from build123d import *

# Parameters (mm, degrees)
F0_W        = 50
F0_H        = 50
F1_DEPTH    = 35
F3_D        = 25
F4_T1_DEPTH = 116.8637576871
F5_T1_DEPTH = 116.8637576871
F6_DEPTH    = 20
F7_T1_DEPTH = 75.7168298797
F10_DEPTH   = 5
F12_DEPTH   = 5


# Not quite as in the source:
# - a fillet or chamfer that OpenCascade refuses, or shapes differently, is made with other operations: its cross-section is extruded or revolved along the edge and cut away or added
# - two fillets or chamfers of one size are made in one step


with BuildPart() as f1:
    # F0 (on Top) → F1 (new body)
    with BuildSketch(Plane.XY):
        with Locations((25, 25)):
            Rectangle(F0_W, F0_H)
    extrude(amount=F1_DEPTH)

    # F3 (through all)
    with Locations(Plane.XZ):
        with Locations((25, 21.1336053908)):
            Hole(F3_D / 2)

    # F4: chamfer of 13 on 1 edges, made by hand

    # F4_s2 → F4_t1 (cut)
    with BuildSketch(Plane.YZ.offset(-33.4318788436)):
        Polygon((0, 22), (13, 35), (0, 35), align=None)
    extrude(amount=F4_T1_DEPTH, mode=Mode.SUBTRACT)

    # F5: chamfer of 13 on 1 edges, made by hand

    # F5_s2 → F5_t1 (cut)
    with BuildSketch(Plane.YZ.offset(-33.4318788436)):
        Polygon((37, 35), (50, 22), (50, 35), align=None)
    extrude(amount=F5_T1_DEPTH, mode=Mode.SUBTRACT)

    # F6 (add): a face of the model
    f6_faces = [f1.faces().sort_by_distance(p)[0] for p in [
        (25, 25, 35),
    ]]
    extrude(f6_faces, amount=F6_DEPTH)

    # F7: chamfer of 5 on 4 edges, made by hand

    # F7_s2 → F7_t1 (cut)
    with BuildSketch(Plane.YZ.offset(-12.8584149398)):
        Polygon((13, 50), (18, 55), (13, 55), align=None)
        Polygon((37, 50), (32, 55), (37, 55), align=None)
    extrude(amount=F7_T1_DEPTH, mode=Mode.SUBTRACT)

    # F9 (on face) → F10 (join)
    with BuildSketch(Plane.YZ.offset(50)):
        Polygon((13, 50), (13, 35), (37, 35), (37, 50), (32, 55), (18, 55), align=None)
    extrude(amount=F10_DEPTH)

    # F11 (on face) → F12 (join)
    with BuildSketch(Plane(origin=(0, 0, 0), x_dir=(0, -1, 0), z_dir=(-1, 0, 0))):
        Polygon((-37, 50), (-37, 35), (-13, 35), (-13, 50), (-18, 55), (-32, 55), align=None)
    extrude(amount=F12_DEPTH)


solid = f1.part
Verification items for the finished model (mm, model axes). A direction names the side the tool comes from. Coordinates: 2 decimals unless noted, no trailing zeros. Write each loop counter-clockwise with the first axis right and the second up, starting at its lowest first coordinate (ties: lowest second). Pieces come first, ordered by that corner, then holes. Notation, with made-up numbers: (-25.5, -21) -> (-4.5, -21) arc R20 ccw to (-4.5, -12) -> close; hole circle Ø4 at (43.5, -31.5). An arc over 180 degrees is marked (long way). One line per item, written item: value. Start each with the question number.
Q1. Mould release check, pull along X, two halves, no side actions. Record for faces 1 (the flat face through (25, 38, 34)), 2 (the flat face through (55, 25, 45)), 3 (the cylindrical face through (28, 25, 9)): pulls with the +X half, pulls with the -X half, needs draft (parallel to the pull), parting line crosses it, or undercut.
Q2. Cross-section at C-C on y = 30. Enter the section's corners in (x, z).
Q3. Cross-section at B-B on x = 25. Enter the section's corners in (y, z).
Q4. Go/stop test with flat-tipped pins: P1, Ø4.5, axis at x = 38.5, z = 41, coming from the -Y side; P2, Ø10.5, axis at y = 13.5, z = 23, coming from the +X side; P3, Ø4, axis at x = 53, y = 27.5, coming from the -Z side; P4, Ø20, axis at x = 25, z = 21.13, coming from the -Y side. Record where each tip stops, or that it passes through.
Q5. Cross-section at A-A on z = 15.5. Enter the section's corners in (x, y), and give its area (3 significant figures).
Q6. Access from +Z, -Z, +X, -X, +Y, -Y to the whole of each face (thin tool, end or side, straight path). Record for faces 4 (the flat face through (25, 13, 42)), 5 (the flat face through (50, 25, 17)), 6 (the flat face through (25, 37, 43)).
Q7. Cross-section at D-D on x = 42. Enter the section's corners in (y, z), and give its area (3 significant figures).
Q8. Thickness scan on L1, parallel to Z at x = 25, y = 28; L2, parallel to X at y = 43, z = 8; L3, parallel to X at y = 14, z = 18. Record the ranges inside material, lowest first. Write a range as from..to.
Checked values:
1. face 1: needs draft
1. face 2: pulls with the +X half
1. face 3: undercut
2. outline: (-5, 35) -> (0, 35) -> (0, 0) -> (50, 0) -> (50, 35) -> (55, 35) -> (55, 55) -> (-5, 55) -> close; hole circle Ø25 at (25, 21.13)
3. outline: (0, 0) -> (50, 0) -> (50, 8.63) -> (0, 8.63) -> close; (11.63, 33.63) -> (38.37, 33.63) -> (37, 35) -> (37, 50) -> (32, 55) -> (18, 55) -> (13, 50) -> (13, 35) -> close
4. P1: stops at y = 13
4. P2: stops at x = 50
4. P3: stops at z = 35
4. P4: passes through
5. outline: (0, 0) -> (13.84, 0) -> (13.84, 50) -> (0, 50) -> close; (36.16, 0) -> (50, 0) -> (50, 50) -> (36.16, 50) -> close
5. area: 1,380 mm²
6. face 4: +Z, +X, -X, -Y
6. face 5: -Z, +X, +Y, -Y
6. face 6: +Z, +X, -X, +Y
7. outline: (0, 0) -> (50, 0) -> (50, 22) -> (37, 35) -> (37, 50) -> (32, 55) -> (18, 55) -> (13, 50) -> (13, 35) -> (0, 22) -> close
7. area: 2,040 mm²
8. L1: z = 0..8.63, 33.63..55
8. L2: x = 0..50
8. L3: x = 0..12.9, 37.1..50
